```python
from build123d import *

# Parameters (mm, degrees)
F1_DEPTH = 12
F2_R     = 1.65
F3_DEPTH = 27.5381246112
F4_R     = 1.65
F5_DEPTH = 17.26183437
F6_R     = 3


# Not quite as in the source:
# - a feature names something its author has since deleted; it is built from what else it names


with BuildPart() as f1:
    # F0 (on Top) → F1 (new body)
    with BuildSketch(Plane.XY):
        Polygon((-22.9726818199, 5.7206649829), (-22.9726818199, 1.1206649829), (-1.5669824788, 1.1206649829), (0.8286588168, 1.1206649829), (2.734780124, 3.6984730734), (0, 5.7206649829), align=None)
        Polygon((2.734780124, 3.6984730734), (0.8286588168, 1.1206649829), (0, 0), (15.6067412389, -11.5401693871), (18.3798691562, -7.870052011), align=None)
        Polygon((0.8286588168, 1.1206649829), (-1.5669824788, 1.1206649829), (0, 0), align=None)
    extrude(amount=F1_DEPTH)

    # F2 (on face) → F3 (cut, through all)
    with BuildSketch(Plane(origin=(2.734780124, 3.6984730734, 0), x_dir=(-0.8040591029, 0.5945493747, 0), z_dir=(0.5945493747, 0.8040591029, 0))):
        with Locations((-7.5987822114, 6)):
            Circle(F2_R)
    extrude(amount=-F3_DEPTH, mode=Mode.SUBTRACT)

    # F4 (on face) → F5 (cut, through all)
    with BuildSketch(Plane(origin=(0, 5.7206649829, 0), x_dir=(-1, 0, 0), z_dir=(0, 1, 0))):
        with Locations((12.9726818199, 6)):
            Circle(F4_R)
    extrude(amount=-F5_DEPTH, mode=Mode.SUBTRACT)

    # F6
    f6_edges = [f1.edges().sort_by_distance(p)[0] for p in [
        (-22.972682, 3.420665, 12),
        (-22.972682, 3.420665, 0),
        (16.993305, -9.705111, 0),
        (16.993305, -9.705111, 12),
    ]]
    fillet(f6_edges, radius=F6_R)


solid = f1.part
```
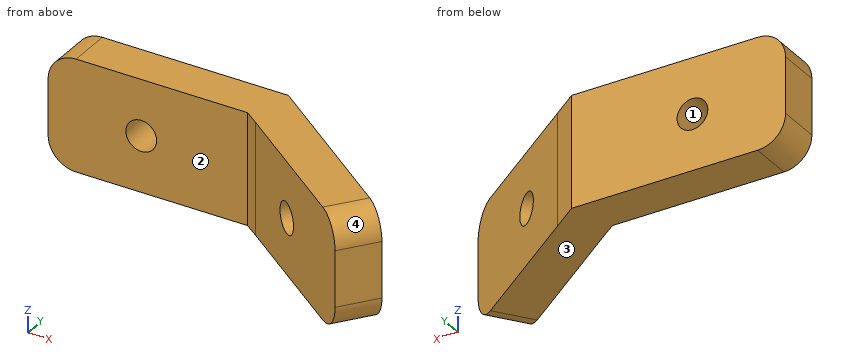
The listing builds one solid part. Answer for the finished solid, in the listing's coordinates (mm). Face numbers are marked on the shaded views. Coordinates: 2 decimals unless noted, no trailing zeros. Loops run counter-clockwise (first coordinate to the right, second up) from the corner with the lowest first, then second, coordinate; pieces in that order, holes last. Notation, with made-up numbers: M 5,60 L 11,60 A17 ccw 11,79 Z; hole C 21.5,-39 d1. An arc over 180 degrees is marked long. Answer as a JSON object with one key per item and string values. Group by question number.
Item 1: Section B-B (z = 11.25) is taken. Write down the section's boundary in (x, y).
Item 2: Section C-C (z = 2.5) is taken. Write down the section's boundary in (x, y), and give its area (3 significant figures).
Item 3: Consider L1, parallel to Z at x = -13, y = 2; L2, parallel to Y at x = -5, z = 2.5; L3, parallel to Z at x = 7, y = -0.75. Determine where each line is inside the solid, lowest interval first.
Item 4: Determine the mould class of the marked faces 1, 2, 3 and 4 for opening direction Z: +Z half, -Z half, draft (parallel to the pull), parting line (faces both ways), or undercut.
Item 5: Section A-A (z = 6) is taken. Write down the section's boundary in (x, y), and give its area (3 significant figures).
Item 6: Each of these flat-tipped pins is pushed along its axis until it touches: P1, Ø4, axis at y = -5, z = 9, coming from the -X side; P2, Ø3, axis at x = 12.5, z = 7.5, coming from the -Y side; P3, Ø2, axis at y = 4, z = 1.5, coming from the +X side. Where does it stop, or does it pass through?
Solved:
{
 "1": {"outline": "M -21.96,1.12 L -1.57,1.12 L 0,0 L 14.79,-10.94 L 17.56,-7.27 L 0,5.72 L -21.96,5.72 Z"},
 "2": {"outline": "M -22.93,1.12 L -1.57,1.12 L 0,0 L 15.57,-11.52 L 18.35,-7.85 L 0,5.72 L -22.93,5.72 Z", "area": "203 mm2"},
 "3": {"L1": "z = 0 to 4.35, 7.65 to 12", "L2": "y = 1.12 to 5.72", "L3": "z = 0 to 5.37, 6.63 to 12"},
 "4": {"face 1": "undercut", "face 2": "draft", "face 3": "-Z half", "face 4": "+Z half"},
 "5": {"outline": "M -22.97,1.12 L -14.62,1.12 L -14.62,5.72 L -22.97,5.72 Z; M -11.32,1.12 L -1.57,1.12 L 0,0 L 4.78,-3.54 L 7.52,0.16 L 0,5.72 L -11.32,5.72 Z; M 7.44,-5.5 L 15.61,-11.54 L 18.38,-7.87 L 10.17,-1.8 Z", "area": "173 mm2"},
 "6": {"P1": "stops at x = 4.06", "P2": "stops at y = -10.35", "P3": "stops at x = 3.68"}
}
